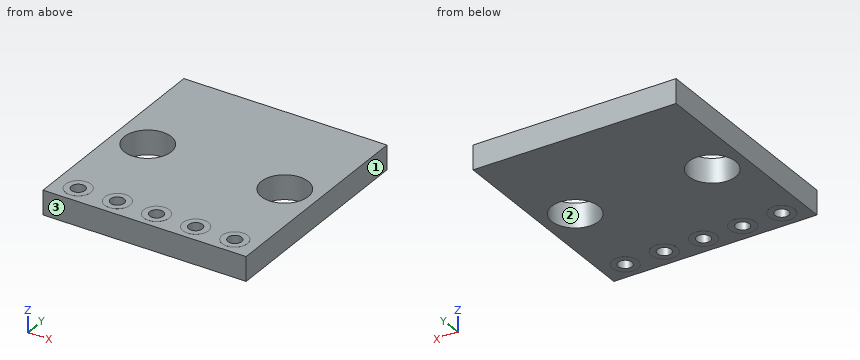
Autodesk Inventor part; units mm, degrees
ref_plane "YZ Plane" through (0, 0, 0) normal (1, 0, 0) x (0, 1, 0)
ref_plane "XZ Plane" through (0, 0, 0) normal (0, 1, 0) x (-1, 0, 0)
ref_plane "XY Plane" through (0, 0, 0) normal (0, 0, 1) x (1, 0, 0)
sketch "Sketch1" plane through (0, 0, 0) normal (0, 0, 1) x (1, 0, 0)
  line L0 (6.5913, -7.112) -> (-6.5913, -7.112)
  line L1 (-6.5913, -7.112) -> (-6.5913, 7.112)
  line L2 (-6.5913, 7.112) -> (6.5913, 7.112)
  line L3 (6.5913, 7.112) -> (6.5913, -7.112)
  line L4 (6.5913, -7.112) -> (-6.5913, 7.112) construction
  line L5 (-6.5913, -7.112) -> (6.5913, 7.112) construction
  point P0 (0, 0)
  dimension "d0" = 13.1826
  dimension "d1" = 14.224
extrude "Extrusion1" add sketch "Sketch1" along normal mid plane 1.5748
sketch "Sketch2" plane through (0, 0, 0.7874) normal (0, 0, 1) x (1, 0, 0)
  circle A0 centre (-4.445, 0.127) radius 1.524
  circle A1 centre (4.445, 0.127) radius 1.524
  line L0 (0, 0) -> (0, 7.112) construction
  line L1 (6.5913, 7.112) -> (-6.5913, 7.112) construction
  dimension "d4" = 3.048
  dimension "d5" = 8.89
  dimension "d6" = 6.985
extrude "Extrusion2" cut sketch "Sketch2" against normal through all
sketch "Sketch3" plane through (0, 0, 0.7874) normal (0, 0, 1) x (1, 0, 0)
  circle A0 centre (0, -5.9055) radius 0.8255 construction
  line L0 (0, -6.731) -> (0, -7.112) construction
  line L1 (6.5913, -7.112) -> (-6.5913, -7.112) construction
  circle A1 centre (-5.08, -5.9055) radius 0.8255
  circle A2 centre (-2.54, -5.9055) radius 0.8255
  circle A3 centre (0, -5.9055) radius 0.8255
  circle A4 centre (2.54, -5.9055) radius 0.8255
  circle A5 centre (5.08, -5.9055) radius 0.8255
  point P0 (0, 0)
  dimension "d9" = 1.651
  dimension "d10" = 0.381
  dimension "d11" = 5.08
  dimension "d14" = 2.54
extrude "Extrusion3" add sketch "Sketch3" along normal blind 0.0025
mirror "Mirror1" about plane through (0, 0, 0) normal (0, 0, 1) of "Extrusion3"
sketch "Sketch4" plane through (-5.08, -5.9055, 0.7899) normal (0, 0, 1) x (1, 0, 0)
  circle A0 centre (0, 0) radius 0.8255 construction
  circle A1 centre (0, 0) radius 0.4445
  circle A2 centre (2.54, 0) radius 0.8255 construction
  line L0 (-1.5113, -1.2065) -> (11.6713, -1.2065) construction
  circle A3 centre (2.54, 0) radius 0.4445
  circle A4 centre (5.08, 0) radius 0.4445
  circle A5 centre (7.62, 0) radius 0.4445
  circle A6 centre (10.16, 0) radius 0.4445
  point P0 (5.08, 5.9055)
  dimension "d21" = 0.889
  dimension "d22" = 2.54
  dimension "d25" = 2.54
extrude "Extrusion4" cut sketch "Sketch4" against normal through all
sketch "Sketch5" plane through (0, 0, 0.7874) normal (0, 0, 1) x (1, 0, 0)
  point P0 (0, 0)
equation "\"d25\" = d22"
properties part number "pcb"
Design review of the part built by this model. Coordinates are the model's own, in mm. Face numbers are marked on the shaded views. Coordinates: 2 decimals unless noted, no trailing zeros. Order: outer loops, then holes, each group sorted by start corner. A loop starts at its lowest first (then second) coordinate and runs counter-clockwise, first axis right, second up.
Item 1: Take a section at D-D, the plane x = -5.08. Count the separate pieces of the cut face and the enclosed holes in it, then the cut area to 3 significant figures.
Item 2: For line 1 (Y direction, x = 0, z = 0.35); line 2 (Y direction, x = 5.25, z = 0.05); line 3 (X direction, y = -5.75, z = -0.4), list the stretches that pass through material, from the lowest coordinate up.
Item 3: Take a section at C-C, the plane z = 0.5. Write out the cut boundary in (x, y) (1 decimal), then the cut area to 3 significant figures.
Item 4: For pin 1 Ø3 at (x, y) = (4, 2.5) entering from -Z; pin 2 Ø4 at (x, y) = (4.5, 0.5) entering from +Z, all flat-tipped, find the tip position at first contact; note any pin that passes through.
Item 5: The part is to be moulded in two halves that separate along Y. For the marked faces 1, 2 and 3, say which applies: pulls with the +Y half, pulls with the -Y half, needs draft (parallel to the pull), parting line crosses it, or undercut.
Item 6: Take a section at A-A, the plane y = -0.5. Write out the cut boundary in (x, z), then the cut area to 3 significant figures.
The answers:
1. separate pieces: 3
1. enclosed holes: 0
1. area: 16.6 mm2
2. line 1: y = -7.11 to -6.35, -5.46 to 7.11
2. line 2: y = -7.11 to -6.32, -5.49 to -1.17, 1.42 to 7.11
2. line 3: x = -6.59 to -5.5, -4.66 to -2.96, -2.12 to -0.42, 0.42 to 2.12, 2.96 to 4.66, 5.5 to 6.59
3. outline: (-6.6, -7.1) - (6.6, -7.1) - (6.6, 7.1) - (-6.6, 7.1) - close; hole circle Ø3 at (-4.4, 0.1); hole circle Ø0.9 at (-5.1, -5.9); hole circle Ø0.9 at (-2.5, -5.9); hole circle Ø0.9 at (0, -5.9); hole circle Ø0.9 at (2.5, -5.9); hole circle Ø3 at (4.4, 0.1); hole circle Ø0.9 at (5.1, -5.9)
3. area: 170 mm2
4. pin 1: stops at z = -0.79
4. pin 2: stops at z = 0.79
5. face 1: needs draft
5. face 2: undercut
5. face 3: pulls with the -Y half
6. outline: (-6.59, -0.79) - (-5.83, -0.79) - (-5.83, 0.79) - (-6.59, 0.79) - close; (-3.06, -0.79) - (3.06, -0.79) - (3.06, 0.79) - (-3.06, 0.79) - close; (5.83, -0.79) - (6.59, -0.79) - (6.59, 0.79) - (5.83, 0.79) - close
6. area: 12.0 mm2
